Read the model definition and answer for the solid it produces. Units are mm, in the model's axes. Face numbers are marked on the shaded views. A direction names the side the tool comes from. Coordinates: 2 decimals unless noted, no trailing zeros. Write each loop counter-clockwise with the first axis right and the second up, starting at its lowest first coordinate (ties: lowest second). Pieces come first, ordered by that corner, then holes.
1) Find the intervals of material crossed by line 1 (X direction, y = 140, z = 11.25); line 2 (Y direction, x = -15, z = 14.5); line 3 (X direction, y = 164, z = 15.5), in increasing order.
2) The part is cut by section A-A (z = 14). Give the number of separate pieces and of enclosed holes in the cut face, then the cut area to 3 significant figures.
3) The part is cut by section D-D (y = 129). Determine the outline of the cut face in (x, z).
4) Which of the six approach directions +Z, -Z, +X, -X, +Y, -Y give full straight-line access (tool end or side, diameter ignored) to the marked faces 4, 5 and 6?
5) The part is cut by section B-B (x = 24). Determine the outline of the cut face in (y, z) (3 decimals).
6) Each of these flat-tipped pins is pushed along its axis until it touches: pin 1 Ø3 at (x, y) = (-15, 140) entering from -Z; pin 2 Ø6 at (y, z) = (166.5, 16.5) entering from -X; pin 3 Ø8 at (y, z) = (159, 11) entering from -X; pin 4 Ø5 at (x, z) = (-30.5, 4) entering from +Y. Where does it stop, or does it pass through?
7) Determine the mould class of the marked faces 1, 2 and 3 for opening direction X: +X half, -X half, draft (parallel to the pull), parting line (faces both ways), or undercut.
8) The part is cut by section C-C (x = -15). Determine the outline of the cut face in (y, z).
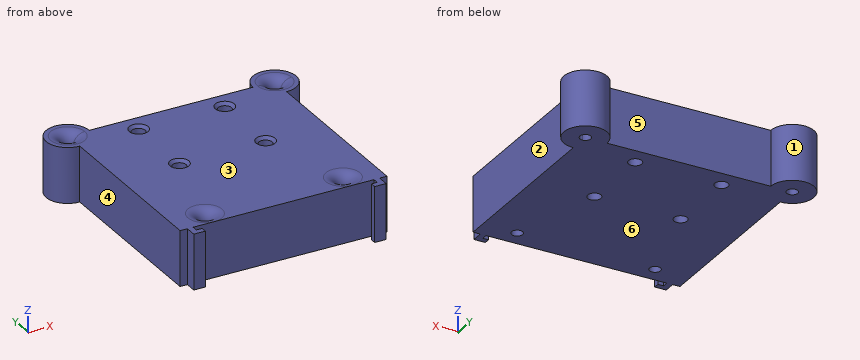
from build123d import *

# Parameters (mm, degrees)
F0_R     = 2.3125
F0_R_2   = 1.925
F1_DEPTH = 19.25
F2_R     = 4
F3_SIZE  = 1


with BuildPart() as f1:
    # F0 (on Top) → F1 (new body)
    with BuildSketch(Plane.XY):
        with BuildLine():
            Line((33.6678512394, 101.9999980927), (36, 101.9999980927))
            Line((36, 101.9999980927), (36, 164.4999980927))
            ThreePointArc((36, 164.4999980927), (30.6966991411, 166.6966972338), (28.5, 171.9999980927))
            Line((28.5, 171.9999980927), (0, 171.9999980927))
            Line((0, 171.9999980927), (0, 101.9999980927))
            Line((0, 101.9999980927), (31.2678519189, 101.9999980927))
            Line((31.2678519189, 101.9999980927), (31.4678515792, 101.9999980927))
            Line((31.4678515792, 101.9999980927), (33.4678515792, 101.9999980927))
            Line((33.4678515792, 101.9999980927), (33.6678512394, 101.9999980927))
        make_face()
        with Locations((15, 139.9999980927)):
            Circle(F0_R, mode=Mode.SUBTRACT)
        with Locations((24, 107.9999980927)):
            Circle(F0_R_2, mode=Mode.SUBTRACT)
        with Locations((15, 165.3999980927)):
            Circle(F0_R, mode=Mode.SUBTRACT)
        with BuildLine():
            Line((0, 101.9999980927), (0, 171.9999980927))
            Line((0, 171.9999980927), (-28.5, 171.9999980927))
            ThreePointArc((-28.5, 171.9999980927), (-30.6966991411, 166.6966972338), (-36, 164.4999980927))
            Line((-36, 164.4999980927), (-36, 101.9999980927))
            Line((-36, 101.9999980927), (-33.6678512394, 101.9999980927))
            Line((-33.6678512394, 101.9999980927), (-33.4678515792, 101.9999980927))
            Line((-33.4678515792, 101.9999980927), (-31.4678515792, 101.9999980927))
            Line((-31.4678515792, 101.9999980927), (-31.2678519189, 101.9999980927))
            Line((-31.2678519189, 101.9999980927), (0, 101.9999980927))
        make_face()
        with Locations((-24, 107.9999980927)):
            Circle(F0_R_2, mode=Mode.SUBTRACT)
        with Locations((-15, 139.9999980927)):
            Circle(F0_R, mode=Mode.SUBTRACT)
        with Locations((-15, 165.3999980927)):
            Circle(F0_R, mode=Mode.SUBTRACT)
        Polygon((-31.4678515792, 99.9999980927), (-31.4678515792, 101.9999980927), (-33.4678515792, 101.9999980927), (-33.4678515792, 97.9999980927), (-29.4678515792, 97.9999980927), (-29.4678515792, 99.9999980927), align=None)
        Polygon((33.4678515792, 97.9999980927), (33.4678515792, 101.9999980927), (31.4678515792, 101.9999980927), (31.4678515792, 99.9999980927), (29.4678515792, 99.9999980927), (29.4678515792, 97.9999980927), align=None)
        with BuildLine():
            ThreePointArc((-36, 164.4999980927), (-30.6966991411, 166.6966972338), (-28.5, 171.9999980927))
            Line((-28.5, 171.9999980927), (-34.075, 171.9999980927))
            ThreePointArc((-34.075, 171.9999980927), (-34.6388194462, 170.6388175389), (-36, 170.0749980927))
            Line((-36, 170.0749980927), (-36, 164.4999980927))
        make_face()
        with BuildLine():
            Line((-34.075, 171.9999980927), (-28.5, 171.9999980927))
            ThreePointArc((-28.5, 171.9999980927), (-41.3033008589, 177.3032989516), (-36, 164.4999980927))
            Line((-36, 164.4999980927), (-36, 170.0749980927))
            ThreePointArc((-36, 170.0749980927), (-37.3611805538, 173.3611786464), (-34.075, 171.9999980927))
        make_face()
        with BuildLine():
            Line((36, 170.0749980927), (36, 164.4999980927))
            ThreePointArc((36, 164.4999980927), (41.3033008589, 166.6966972338), (43.5, 171.9999980927))
            ThreePointArc((43.5, 171.9999980927), (36, 179.4999980927), (28.5, 171.9999980927))
            Line((28.5, 171.9999980927), (34.075, 171.9999980927))
            ThreePointArc((34.075, 171.9999980927), (36, 173.9249980927), (37.925, 171.9999980927))
            ThreePointArc((37.925, 171.9999980927), (37.3611805538, 170.6388175389), (36, 170.0749980927))
        make_face()
        with BuildLine():
            ThreePointArc((28.5, 171.9999980927), (30.6966991411, 166.6966972338), (36, 164.4999980927))
            Line((36, 164.4999980927), (36, 170.0749980927))
            ThreePointArc((36, 170.0749980927), (34.6388194462, 170.6388175389), (34.075, 171.9999980927))
            Line((34.075, 171.9999980927), (28.5, 171.9999980927))
        make_face()
    extrude(amount=F1_DEPTH)

    # F2
    f2_edges = [f1.edges().sort_by_distance(p)[0] for p in [
        (-36, 173.924998, 19.25),
        (-25.925, 107.999998, 19.25),
        (22.075, 107.999998, 19.25),
        (37.925, 171.999998, 19.25),
    ]]
    fillet(f2_edges, radius=F2_R)

    # F3
    f3_edges = [f1.edges().sort_by_distance(p)[0] for p in [
        (-17.3125, 165.399998, 19.25),
        (-17.3125, 139.999998, 19.25),
        (12.6875, 139.999998, 19.25),
        (12.6875, 165.399998, 19.25),
    ]]
    chamfer(f3_edges, length=F3_SIZE)


solid = f1.part
Reported:
1. line 1: x = -36 to -17.31, -12.69 to 12.69, 17.31 to 36
1. line 2: y = 102 to 137.69, 142.31 to 163.09, 167.71 to 172
1. line 3: x = -36 to -16.84, -13.16 to 13.16, 16.84 to 36
2. separate pieces: 1
2. enclosed holes: 8
2. area: 5,220 mm2
3. outline: (-36, 0) - (36, 0) - (36, 19.25) - (-36, 19.25) - close
4. face 4: +Z, -Z, -X, -Y
4. face 5: +Z, -Z, +Y
4. face 6: -Z, +X, -X, +Y, -Y
5. outline: (102, 0) - (106.075, 0) - (106.075, 15.25) arc R4 ccw to (102.075, 19.25) - (102, 19.25) - close; (109.925, 0) - (172, 0) - (172, 19.25) - (113.925, 19.25) arc R4 ccw to (109.925, 15.25) - close
6. pin 1: passes through
6. pin 2: stops at x = -43.07
6. pin 3: stops at x = -36
6. pin 4: stops at y = 178.87
7. face 1: undercut
7. face 2: +X half
7. face 3: draft
8. outline: (102, 0) - (137.69, 0) - (137.69, 18.25) - (136.69, 19.25) - (102, 19.25) - close; (142.31, 0) - (163.09, 0) - (163.09, 18.25) - (162.09, 19.25) - (143.31, 19.25) - (142.31, 18.25) - close; (167.71, 0) - (172, 0) - (172, 19.25) - (168.71, 19.25) - (167.71, 18.25) - close
